Read the model definition and answer for the solid it produces. Units are mm, in the model's axes. A direction names the side the tool comes from. Coordinates: 2 decimals unless noted, no trailing zeros. Loops run counter-clockwise (first coordinate to the right, second up) from the corner with the lowest first, then second, coordinate; pieces in that order, holes last.
Q1. Which of the six approach directions +Z, -Z, +X, -X, +Y, -Y give full straight-line access (tool end or side, diameter ignored) to faces 5 (the face through (-1, 2, 2.5)), 6 (the face through (2, 4, 1)), 7 (the face through (-2, 3, -1))?
Q2. The mould has two halves that part along X. Classify faces 1 (the face through (1, 4, -1)), 2 (the face through (1, 2, -2.5)), 3 (the face through (-0.709, 3.472, 1.163)), 4 (the face through (-3, 2, 1)): pulls with the +X half, pulls with the -X half, needs draft (parallel to the pull), parting line crosses it, or undercut.
Q3. Section C-C (z = -0.65) is taken. Give the vertices of the cut face in (x, y), then the cut area to 3 significant figures.
Q4. A flat-ended cylindrical pin translates along its axis: P1, Ø3.5, axis at x = 2, y = 4.5, coming from the +Z side. Find the tip coordinate at first contact, or state that the pin passes through.
Q5. Section B-B (y = 1.1) is taken. Give the vertices of the cut face in (x, z), then the cut area to 3 significant figures.
Q6. Straight lines are drawn through the part: line 1 (X direction, y = 3, z = 1.4); line 2 (Z direction, x = -2.65, y = 0.5); line 3 (Z direction, x = 1.7, y = 3.35). For each, find the intervals that lie inside material, in ascending order.
Q7. Section D-D (x = -1.05) is taken. Give the vertices of the cut face in (y, z).
Q8. Section A-A (y = 4.8) is taken. Give the vertices of the cut face in (x, z).
from build123d import *

# Parameters (mm, degrees)
SKETCH1_W           = 6
SKETCH1_H           = 5
BOSS_EXTRUDE1_DEPTH = 6
CUT_EXTRUDE1_DEPTH  = 3.5
CUT_EXTRUDE2_DEPTH  = 1.5
CUT_EXTRUDE3_DEPTH  = 3.5
CUT_EXTRUDE4_DEPTH  = 1.5


with BuildPart() as part:
    # Sketch1 → Boss-Extrude1 (new body)
    with BuildSketch(Plane(origin=(0, 0, 0), x_dir=(1, 0, 0), z_dir=(0, 1, 0))):
        Rectangle(SKETCH1_W, SKETCH1_H)
    extrude(amount=BOSS_EXTRUDE1_DEPTH)

    # Sketch2 → Cut-Extrude1 (cut)
    with BuildSketch(Plane.XY.offset(2.5)):
        Polygon((-3, 5), (0, 3), (0, 6), (-3, 6), align=None)
    extrude(amount=-CUT_EXTRUDE1_DEPTH, mode=Mode.SUBTRACT)

    # Sketch4 → Cut-Extrude2 (cut)
    with BuildSketch(Plane.XY.offset(2.5)):
        Polygon((0, 3), (3, 1), (3, 6), (0, 6), align=None)
    extrude(amount=-CUT_EXTRUDE2_DEPTH, mode=Mode.SUBTRACT)

    # Sketch5 → Cut-Extrude3 (cut)
    with BuildSketch(Plane(origin=(0, 0, -2.5), x_dir=(-1, 0, 0), z_dir=(0, 0, -1))):
        Polygon((0, 6), (-3, 6), (0, 3), align=None)
    extrude(amount=-CUT_EXTRUDE3_DEPTH, mode=Mode.SUBTRACT)

    # Sketch6 → Cut-Extrude4 (cut)
    with BuildSketch(Plane(origin=(0, 0, -2.5), x_dir=(-1, 0, 0), z_dir=(0, 0, -1))):
        Polygon((0, 3), (3, 0), (3, 6), (0, 6), align=None)
    extrude(amount=-CUT_EXTRUDE4_DEPTH, mode=Mode.SUBTRACT)


solid = part.part
Numbers:
1. face 5: +Z, +X, -X, +Y, -Y
1. face 6: +Z, +X, +Y
1. face 7: -Z, -X, +Y
2. face 1: undercut
2. face 2: needs draft
2. face 3: undercut
2. face 4: pulls with the -X half
3. outline: (-3, 0) - (3, 0) - (3, 6) - (0, 3) - (-3, 5) - close
3. area: 25.5 mm2
4. P1: stops at z = 1
5. outline: (-3, -1) - (-1.9, -1) - (-1.9, -2.5) - (3, -2.5) - (3, 1) - (2.85, 1) - (2.85, 2.5) - (-3, 2.5) - close
5. area: 28.1 mm2
6. line 1: x = -3 to 0
6. line 2: z = -1 to 2.5
6. line 3: z = -2.5 to 1
7. outline: (0, -2.5) - (1.95, -2.5) - (1.95, -1) - (3.7, -1) - (3.7, 2.5) - (0, 2.5) - close
8. outline: (-3, -1) - (-2.7, -1) - (-2.7, 2.5) - (-3, 2.5) - close; (1.8, -2.5) - (3, -2.5) - (3, 1) - (1.8, 1) - close
